```python
from build123d import *

# Parameters (mm, degrees)
CROQUIS1_R              = 70
SALIENTE_EXTRUIR1_DEPTH = 10
CROQUIS4_R              = 47.5
SALIENTE_EXTRUIR2_DEPTH = 22
MATRIZC1_COUNT          = 6


with BuildPart() as part:
    # Croquis1 → Saliente-Extruir1 (new body)
    with BuildSketch(Plane(origin=(0, 0, 0), x_dir=(1, 0, 0), z_dir=(0, 1, 0))):
        with Locations(Location((0, 0, 0), (0, 0, 270))):
            Circle(CROQUIS1_R)
    extrude(amount=SALIENTE_EXTRUIR1_DEPTH)

    # Croquis4 → Saliente-Extruir2 (add)
    with BuildSketch(Plane(origin=(0, 0, 0), x_dir=(-1, 0, 0), z_dir=(0, -1, 0))):
        with Locations(Location((0, 0, 0), (0, 0, 90))):
            Circle(CROQUIS4_R)
    extrude(amount=SALIENTE_EXTRUIR2_DEPTH)

    # Croquis6 → Taladro roscado M12x1.51 (revolve, cut)
    with BuildSketch(Plane(origin=(60, 10, 0), x_dir=(0, 0, 1), z_dir=(1, 0, 0))):
        Polygon((0, 0), (0, 34.65451825), (5.25, 31.5), (5.25, 0), align=None)
    taladro_roscado_m12x1_51 = revolve(axis=Axis((60, 16.35, 0), (0, -1, 0)), mode=Mode.SUBTRACT)

    # MatrizC1: Taladro roscado M12x1.51 ×6 about axis
    matrizc1_axis = Axis((-0.339409177, 0, 0), (0, 1, 0))
    for i in range(1, MATRIZC1_COUNT):
        add(taladro_roscado_m12x1_51.rotate(matrizc1_axis, i * 360 / MATRIZC1_COUNT), mode=Mode.SUBTRACT)


solid = part.part
```
Input: part model. Units: mm. Frame: model coordinates. A direction names the side the tool comes from. Round coordinates to 2 decimals unless told otherwise and drop trailing zeros. Write each loop counter-clockwise with the first axis right and the second up, starting at its lowest first coordinate (ties: lowest second). Pieces come first, ordered by that corner, then holes. Notation, with made-up numbers: M 38,66.5 L 49,66.5 A26 cw 49,86.5 Z; hole C 54,56.25 d9. An arc over 180 degrees is marked long. Write each question's results on one line, items separated by ' | '.
Q1. Section query A-A (x = 0). Return loops of the section in (y, z).
Results:
outline: M -22,-47.5 L 0,-47.5 L 0,-70 L 10,-70 L 10,70 L 0,70 L 0,47.5 L -22,47.5 Z
Q2. Pin query (flat end, axial travel): P1, Ø6, axis at x = -32.5, y = 1.5, coming from the -Z side; P2, Ø12, axis at x = 60, z = 0, coming from the -Y side; P3, Ø4, axis at y = -4, z = -15.5, coming from the -X side. Return the tip coordinate at first contact, or that it passes through.
Results:
P1: stops at z = -63.48 | P2: stops at y = 0 | P3: stops at x = -45.54
Q3. Draft query along Z for faces 3 (the face through (-46.37, -10.85, 10.3)), 4 (the face through (-55.473, 5.07, 0.683)), 5 (the face through (1, -22, 1)), 6 (the face through (65.125, 5.07, -1.138)). Return one class per face: released by +Z, released by -Z, zero draft, split by the parting line, or undercut.
Results:
face 3: split by the parting line | face 4: undercut | face 5: zero draft | face 6: undercut
Q4. Section query D-D (y = 6.5). Return loops of the section in (x, z), and give its area (3 significant figures).
Results:
outline: C 0,0 d140; hole C -60.68,0 d10.5; hole C -30.51,-52.26 d10.5; hole C -30.51,52.26 d10.5; hole C 29.83,-52.26 d10.5; hole C 29.83,52.26 d10.5; hole C 60,0 d10.5 | area: 14,900 mm^2
Q5. Access query for faces 1 (the face through (33.378, 5.07, 56.125)), 2 (the face through (-15, 0, 46)). Directions: +Z, -Z, +X, -X, +Y, -Y. A direction counts if a zero-diameter tool reaches every point of the face in a straight line with its end or side. Return the directions, or none.
Results:
face 1: +Y, -Y | face 2: -Y
Q6. Section query C-C (x = 60). Return loops of the section in (y, z).
Results:
outline: M 0,-36.06 L 10,-36.06 L 10,-5.25 L 0,-5.25 Z; M 0,5.25 L 10,5.25 L 10,36.06 L 0,36.06 Z
Q7. Section query B-B (z = -18). Return loops of the section in (x, y), and give its area (3 significant figures).
Results:
outline: M -67.65,0 L -43.96,0 L -43.96,-22 L 43.96,-22 L 43.96,0 L 67.65,0 L 67.65,10 L -67.65,10 Z | area: 3,290 mm^2
Q8. Line query: line 1 along X through (y, z) = (7, 0); line 2 along X through (y, z) = (6.5, 55); line 3 along Y through (x, z) = (-60.5, 14). Output: solid intervals per line, ascending.
Results:
line 1: x = -70 to -65.93, -55.43 to 54.75, 65.25 to 70 | line 2: x = -43.3 to -34.98, -26.03 to 25.35, 34.31 to 43.3 | line 3: y = 0 to 10
